Build history of the part. All positions in model axes, mm. Face numbers are marked on the shaded views. Give positions to 0.01 mm unless a question says otherwise; leave off trailing zeros. Order: outer loops, then holes, each group sorted by start corner. A loop starts at its lowest first (then second) coordinate and runs counter-clockwise, first axis right, second up. Notation, with made-up numbers: (57.5, 22) -> (88.5, 22) arc R28 ccw to (88.5, 55) -> close; hole circle Ø4 at (1.25, 8). An arc over 180 degrees is marked (long way). One line per item, written item: value. Start each with the question number.
(1) Saw through at D-D on z = 39. Give the cut face in (x, y).
(2) Saw through at B-B on x = 16. Give the cut face in (y, z), plus the area to 3 significant figures.
(3) Two-plate mould, pull along Y, no slides. Class the marked faces 1, 2, 3 and 4: +Y half, -Y half, draft (parallel to the pull), parting line (faces both ways), or undercut.
(4) Probe line 1 (Z direction, x = 25, y = 23); line 2 (Y direction, x = 12.5, z = 49); line 3 (Z direction, x = 3, y = 17.5). List the from-to ranges inside material, lowest first.
(5) Saw through at A-A on y = 19.5. Give the cut face in (x, z), plus the area to 3 significant figures.
(6) Saw through at C-C on y = 12. Give the cut face in (x, z).
(7) Pin check, flat tips, straight feed: pin 1 (0.9 mm diameter, centred on x = 23, y = 37.5, fed in from -Z); pin 2 (6 mm diameter, centred on x = 9.5, y = 29, fed in from -Z); pin 3 (1.5 mm diameter, centred on x = 33.5, y = 26.5, fed in from -Z). Stop position of each tip, or through.
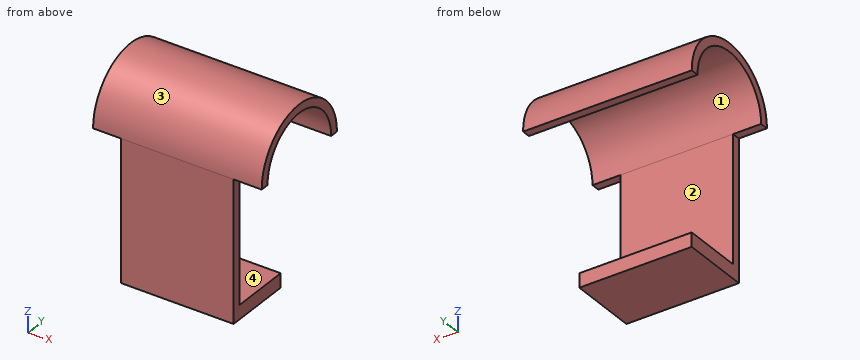
Autodesk Fusion 360 part; units mm, degrees
sketch "Sketch2" plane through (0, 0, 0) normal (0, 0, 1) x (1, 0, 0)
  line L0 (0, 0) -> (40, 0)
  line L1 (40, 0) -> (40, 24.4086)
  line L2 (40, 24.4086) -> (0, 24.4086)
  line L3 (0, 24.4086) -> (0, 0)
extrude "Extrude1" add sketch "Sketch2" along normal blind 5
sketch "Sketch3" plane through (0, 0, 0) normal (0, -1, 0) x (1, 0, 0)
  line L0 (0, 0) -> (40, 0)
  line L1 (40, 0) -> (40, 5)
  line L2 (40, 5) -> (0, 5)
  line L3 (0, 5) -> (0, 0)
  line L4 (0, 0) -> (40, 0)
  line L5 (40, 0) -> (40, 50)
  line L6 (40, 50) -> (0, 50)
  line L7 (0, 50) -> (0, 0)
extrude "Extrude2" add sketch "Sketch3" against normal blind 3 contours L2 L5 L6 L7
sketch "Sketch4" plane through (40, 0, 0) normal (1, 0, 0) x (0, 1, 0)
  line L0 (0, 0) -> (24.4086, 0)
  line L1 (24.4086, 0) -> (24.4086, 5)
  line L2 (24.4086, 5) -> (3, 5)
  line L3 (3, 5) -> (3, 50)
  line L4 (3, 50) -> (0, 50)
  line L5 (0, 50) -> (0, 0)
  line L6 (19.5, 40) -> (19.5, 70) construction
  arc A0 (36, 50) -> (3, 50) centre (19.5, 50) ccw
  arc A1 (39, 50) -> (0, 50) centre (19.5, 50) ccw
  line L7 (36, 50) -> (39, 50)
  line L8 (36, 50) -> (39, 50)
  line L9 (0, 50) -> (3, 50)
  dimension "d7" = 16.5
  dimension "d8" = 3
extrude "Extrude3" add sketch "Sketch4" along normal blind 10 and the other way blind 50 contours L4 A0 A1 L7 L8 L9
equation "d7 = ( 33 / 2 ) * 1 mm"
Results below:
1. outline: (0, 0) -> (40, 0) -> (40, 3) -> (0, 3) -> close
2. outline: (0, 0) -> (24.41, 0) -> (24.41, 5) -> (3, 5) -> (3, 50) arc R16.5 cw to (36, 50) -> (39, 50) arc R19.5 ccw to (0, 50) -> close
2. area: 427 mm²
3. face 1: undercut
3. face 2: +Y half
3. face 3: parting line
3. face 4: draft
4. line 1: z = 0 to 5, 66.12 to 69.18
4. line 2: y = 0 to 3
4. line 3: z = 0 to 5, 66.38 to 69.4
5. outline: (-10, 66.5) -> (50, 66.5) -> (50, 69.5) -> (-10, 69.5) -> close; (0, 0) -> (40, 0) -> (40, 5) -> (0, 5) -> close
5. area: 380 mm²
6. outline: (-10, 64.7) -> (50, 64.7) -> (50, 68) -> (-10, 68) -> close; (0, 0) -> (40, 0) -> (40, 5) -> (0, 5) -> close
7. pin 1: stops at z = 50
7. pin 2: stops at z = 60.77
7. pin 3: stops at z = 64.57
